```python
from build123d import *

# Parameters (mm, degrees)
CHAMFER1_SIZE      = 0.5
CHAMFER2_SIZE      = 0.3
CUT_EXTRUDE1_DEPTH = 2.5
CHAMFER3_SIZE      = 0.3


with BuildPart() as part:
    # Sketch1 → Revolve1 (revolve)
    with BuildSketch(Plane.XY):
        Polygon((0, 0), (0, 2.75), (3, 2.75), (3, 1.49), (23, 1.49), (23, 0), align=None)
    revolve(axis=Axis((-88.705490849, 0, 0), (1, 0, 0)))

    # Chamfer1
    chamfer1_edges = [part.edges().sort_by_distance(p)[0] for p in [
        (23, -1.49, 0),
    ]]
    chamfer(chamfer1_edges, length=CHAMFER1_SIZE)

    # Chamfer2
    chamfer2_edges = [part.edges().sort_by_distance(p)[0] for p in [
        (0, -2.75, 0),
    ]]
    chamfer(chamfer2_edges, length=CHAMFER2_SIZE)

    # Sketch3 → Cut-Extrude1 (cut)
    with BuildSketch(Plane(origin=(0, 0, 0), x_dir=(0, 0, -1), z_dir=(1, 0, 0))):
        Polygon((-1.443375673, 0), (-0.721687836, -1.25), (0.721687836, -1.25), (1.443375673, 0), (0.721687836, 1.25), (-0.721687836, 1.25), align=None)
    extrude(amount=CUT_EXTRUDE1_DEPTH, mode=Mode.SUBTRACT)

    # Chamfer3
    chamfer3_edges = [part.edges().sort_by_distance(p)[0] for p in [
        (0, 0.625, 1.082531755),
        (0, -0.625, 1.082531755),
        (0, -1.25, 0),
        (0, -0.625, -1.082531755),
        (0, 0.625, -1.082531755),
        (0, 1.25, 0),
    ]]
    chamfer(chamfer3_edges, length=CHAMFER3_SIZE)


solid = part.part
```
The listing builds one solid part. Answer for the finished solid, in the listing's coordinates (mm). A direction names the side the tool comes from. Give positions to 0.01 mm unless a question says otherwise; leave off trailing zeros. Order: outer loops, then holes, each group sorted by start corner. A loop starts at its lowest first (then second) coordinate and runs counter-clockwise, first axis right, second up. Notation, with made-up numbers: (24.5, 71) - (53.5, 71) arc R21 cw to (53.5, 90) - close; hole circle Ø4 at (10, -13). An arc over 180 degrees is marked (long way). Use one line per item in the form item = value. Start each with the question number.
(1) The mould has two halves that part along Y. Classify faces 4 (the flat face through (0, -2, 0)), 5 (the cylindrical face through (1.669, -0.596, -2.685)), 6 (the flat face through (1.38, -0.63, -1.08)): released by +Y, released by -Y, zero draft, split by the parting line, or undercut.
(2) For faces 1 (the flat face through (3, 1.2, -1.2)), 2 (the flat face through (23, 0, 0)), 3 (the flat face through (2.5, 0, 0)), determine the directions among +Z, -Z, +X, -X, +Y, -Y from which every point of the face is accessible in a straight line to the end or side of a thin tool.
(3) A cutting plane is placed at A-A, the plane x = 1.5. Write down the section's boundary in (y, z).
(4) Consider line 1 (X direction, y = 1, z = 2.05); line 2 (X direction, y = 0.35, z = -0.55); line 3 (Z direction, x = 4, y = -0.25). Determine where each line is inside the solid, lowest interval first. Write a range as from..to.
(5) A cutting plane is placed at B-B, the plane z = 0. Write down the section's boundary in (x, y), then the cut area to 3 significant figures.
(6) A cutting plane is placed at C-C, the plane x = 13.5. Write down the section's boundary in (y, z).
(7) Flat-ended cylindrical pins translate along their axes: pin 1 Ø2 at (x, z) = (5, 0.5) entering from +Y; pin 2 Ø2 at (y, z) = (0, 0.5) entering from -X; pin 3 Ø1.5 at (x, y) = (17.5, -0.5) entering from -Z. Find the tip coordinate at first contact, or state that the pin passes through.
Ans:
q1.face_4 = zero draft
q1.face_5 = split by the parting line
q1.face_6 = undercut
q2.face_1 = +X
q2.face_2 = +Z, -Z, +X, +Y, -Y
q2.face_3 = -X
q3.outline = circle Ø5.5 at (0, 0); hole (-1.25, -0.72) - (0, -1.44) - (1.25, -0.72) - (1.25, 0.72) - (0, 1.44) - (-1.25, 0.72) - close
q4.line_1 = 0..3
q4.line_2 = 2.5..23
q4.line_3 = -1.47..1.47
q5.outline = (0, -2.45) - (0.3, -2.75) - (3, -2.75) - (3, -1.49) - (22.5, -1.49) - (23, -0.99) - (23, 0.99) - (22.5, 1.49) - (3, 1.49) - (3, 2.75) - (0.3, 2.75) - (0, 2.45) - (0, 1.55) - (0.3, 1.25) - (2.5, 1.25) - (2.5, -1.25) - (0.3, -1.25) - (0, -1.55) - close
q5.area = 69.4 mm^2
q6.outline = circle Ø2.98 at (0, 0)
q7.pin_1 = 1.49
q7.pin_2 = 0.12
q7.pin_3 = -1.49
